Design review of the part shown in the three views and the two pictorial views. Dimensions are in mm from the part's minimum x, y and z. Round coordinates to 2 decimals unless told otherwise and drop trailing zeros. Loops run counter-clockwise (first coordinate to the right, second up) from the corner with the lowest first, then second, coordinate; pieces in that order, holes last. Notation, with made-up numbers: (36.25, 43) - (86.25, 43) arc R25 ccw to (86.25, 82) - close; hole circle Ø9 at (22, -26.75). An arc over 180 degrees is marked (long way). Return JSON: item names as keys, results as strings. Group by question number.
(1) We need section B-B, the plane x = 0.7. Write out the cut boundary in (y, z) (3 decimals).
(2) We need section A-A, the plane y = 3. Write out the cut boundary in (x, z), and give its area (3 significant figures).
(3) Wall thickness on L1, parallel to Z at x = 0.3, y = 3.25; L2, parallel to Z at x = 0.9, y = 7.5; L3, parallel to Z at x = 1.95, y = 14.5: over which ranges is each line inside the solid? List them lowest first. Write a range as [from, to].
(4) We need section D-D, the plane z = 35. Write out the cut boundary in (x, y), and give its area (3 significant figures).
(5) We need section C-C, the plane y = 6.5. Write out the cut boundary in (x, z).
(6) Clearance check with flat-ended pins moving along their axes: pin 1 (1.3 mm diameter, centred on x = 1, z = 48, fed in from -Y); pin 2 (0.8 mm diameter, centred on x = 1, y = 4, fed in from -Z); pin 3 (1.3 mm diameter, centred on x = 1.5, z = 90.5, fed in from +Y) (3 decimals); pin 4 (6 mm diameter, centred on y = 8.5, z = 82, fed in from -X). State where each tip first meets the part, or that it passes through.
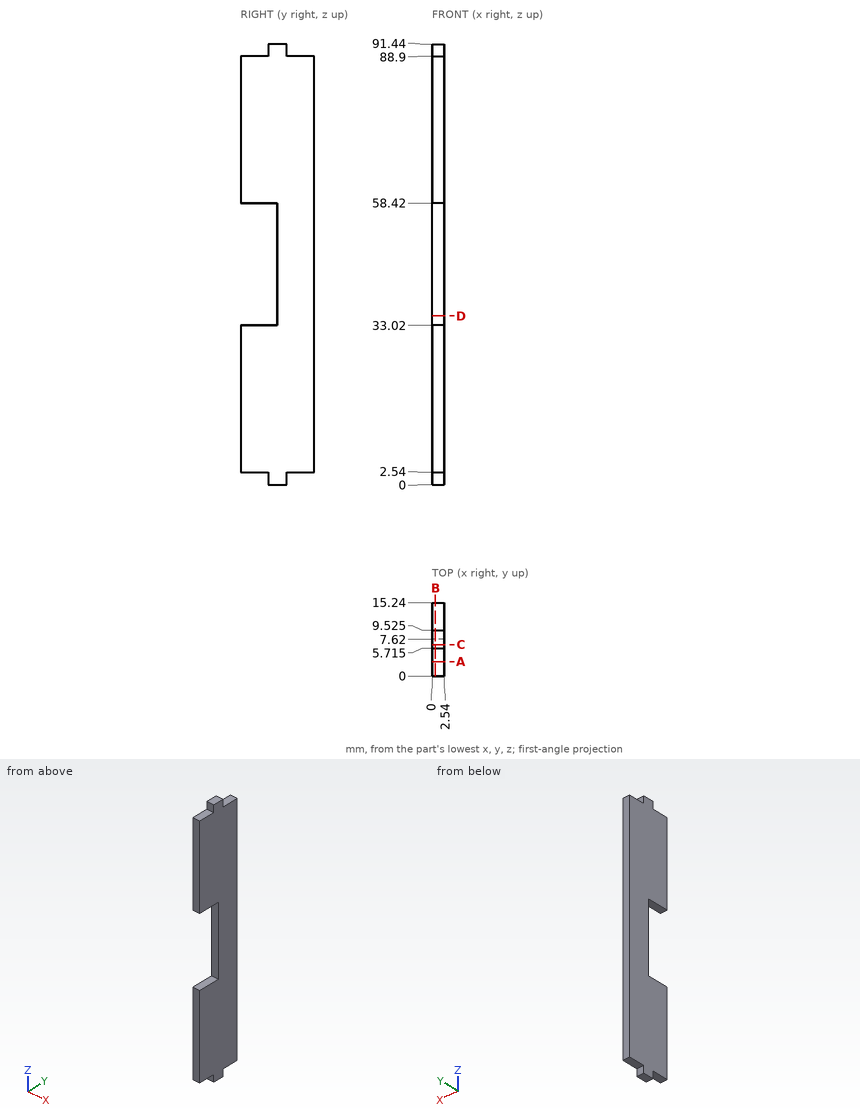
Solutions:
{
 "1": {"outline": "(0, 2.54) - (5.715, 2.54) - (5.715, 0) - (9.525, 0) - (9.525, 2.54) - (15.24, 2.54) - (15.24, 88.9) - (9.525, 88.9) - (9.525, 91.44) - (5.715, 91.44) - (5.715, 88.9) - (0, 88.9) - (0, 58.42) - (7.62, 58.42) - (7.62, 33.02) - (0, 33.02) - close"},
 "2": {"outline": "(0, 2.54) - (2.54, 2.54) - (2.54, 33.02) - (0, 33.02) - close; (0, 58.42) - (2.54, 58.42) - (2.54, 88.9) - (0, 88.9) - close", "area": "155 mm^2"},
 "3": {"L1": "[2.54, 33.02], [58.42, 88.9]", "L2": "[0, 33.02], [58.42, 91.44]", "L3": "[2.54, 88.9]"},
 "4": {"outline": "(0, 7.62) - (2.54, 7.62) - (2.54, 15.24) - (0, 15.24) - close", "area": "19.4 mm^2"},
 "5": {"outline": "(0, 0) - (2.54, 0) - (2.54, 33.02) - (0, 33.02) - close; (0, 58.42) - (2.54, 58.42) - (2.54, 91.44) - (0, 91.44) - close"},
 "6": {"pin 1": "y = 7.62", "pin 2": "z = 2.54", "pin 3": "y = 9.525", "pin 4": "x = 0"}
}
